from build123d import *

# Parameters (mm, degrees)
BOSS_EXTRU_1_DEPTH      = 20
ENL_V_MAT_EXTRU_1_DEPTH = 60.247890258
ESQUISSE5_W             = 53.8
ESQUISSE5_H             = 20
ESQUISSE5_R             = 3.2
ENL_V_MAT_EXTRU_2_DEPTH = 3
ESQUISSE6_W             = 53.8
ESQUISSE6_H             = 20
ESQUISSE6_R             = 6.75
ENL_V_MAT_EXTRU_3_DEPTH = 1.6
ESQUISSE7_W             = 53.8
ESQUISSE7_H             = 20
ENL_V_MAT_EXTRU_4_DEPTH = 3.2
CHANFREIN2_SIZE         = 3


with BuildPart() as part:
    # Esquisse1 → Boss.-Extru.1 (new body)
    with BuildSketch(Plane.XY):
        Polygon((0, 0), (40.1, 0), (40.1, 27.6), (46.95, 27.6), (46.95, 30.1), (40.1, 30.1), (40.1, 35.2), (36.7, 35.2), (36.7, 38.4), (16.402, 38.4), (16.402, 40), (12.852, 40), (12.852, 43), (6.452, 43), (6.452, 40), (2.902, 40), (2.902, 38.4), (0, 38.4), (0, 30.1), (-6.85, 30.1), (-6.85, 27.6), (0, 27.6), align=None)
    extrude(amount=BOSS_EXTRU_1_DEPTH)

    # Esquisse2 → Enlèv. mat.-Extru.1 (cut, through all)
    with BuildSketch(Plane(origin=(0, 30.1, 0), x_dir=(1, 0, 0), z_dir=(0, 1, 0))):
        with BuildLine():
            Line((-6.85, -3.75), (-6.85, -6.25))
            Line((-6.85, -6.25), (-6.186029115, -6.25))
            ThreePointArc((-6.186029115, -6.25), (-2.22, -5), (-6.186029115, -3.75))
            Line((-6.186029115, -3.75), (-6.85, -3.75))
        make_face()
        with BuildLine():
            Line((46.95, -6.25), (46.286029115, -6.25))
            ThreePointArc((46.286029115, -6.25), (42.32, -5), (46.286029115, -3.75))
            Line((46.286029115, -3.75), (46.95, -3.75))
            Line((46.95, -3.75), (46.95, -6.25))
        make_face()
        with BuildLine():
            Line((46.95, -16.25), (46.286029115, -16.25))
            ThreePointArc((46.286029115, -16.25), (42.32, -15), (46.286029115, -13.75))
            Line((46.286029115, -13.75), (46.95, -13.75))
            Line((46.95, -13.75), (46.95, -16.25))
        make_face()
        with BuildLine():
            Line((-6.85, -13.75), (-6.186029115, -13.75))
            ThreePointArc((-6.186029115, -13.75), (-2.22, -15), (-6.186029115, -16.25))
            Line((-6.186029115, -16.25), (-6.85, -16.25))
            Line((-6.85, -16.25), (-6.85, -13.75))
        make_face()
    extrude(amount=-ENL_V_MAT_EXTRU_1_DEPTH, mode=Mode.SUBTRACT)

    # Esquisse5 → Enlèv. mat.-Extru.2 (cut)
    with BuildSketch(Plane(origin=(0, 43, 0), x_dir=(1, 0, 0), z_dir=(0, 1, 0))):
        with Locations((20.05, -10)):
            Rectangle(ESQUISSE5_W, ESQUISSE5_H)
        with Locations(Location((9.652, -10, 0), (0, 0, 180))):
            Circle(ESQUISSE5_R, mode=Mode.SUBTRACT)
    extrude(amount=-ENL_V_MAT_EXTRU_2_DEPTH, mode=Mode.SUBTRACT)

    # Esquisse6 → Enlèv. mat.-Extru.3 (cut)
    with BuildSketch(Plane(origin=(0, 40, 0), x_dir=(1, 0, 0), z_dir=(0, 1, 0))):
        with Locations((20.05, -10)):
            Rectangle(ESQUISSE6_W, ESQUISSE6_H)
        with Locations(Location((9.652, -10, 0), (0, 0, 270))):
            Circle(ESQUISSE6_R, mode=Mode.SUBTRACT)
    extrude(amount=-ENL_V_MAT_EXTRU_3_DEPTH, mode=Mode.SUBTRACT)

    # Esquisse7 → Enlèv. mat.-Extru.4 (cut)
    with BuildSketch(Plane(origin=(0, 38.4, 0), x_dir=(1, 0, 0), z_dir=(0, 1, 0))):
        with Locations((20.05, -10)):
            Rectangle(ESQUISSE7_W, ESQUISSE7_H)
        with BuildLine():
            Line((13.446733192, -18.6), (36.7, -18.6))
            Line((36.7, -18.6), (36.7, -1.4))
            Line((36.7, -1.4), (13.446733192, -1.4))
            ThreePointArc((13.446733192, -1.4), (0.252, -10), (13.446733192, -18.6))
        make_face(mode=Mode.SUBTRACT)
    extrude(amount=-ENL_V_MAT_EXTRU_4_DEPTH, mode=Mode.SUBTRACT)

    # Chanfrein2
    chanfrein2_edges = [part.edges().sort_by_distance(p)[0] for p in [
        (36.7, 38.4, 10),
    ]]
    chamfer(chanfrein2_edges, length=CHANFREIN2_SIZE)


solid = part.part
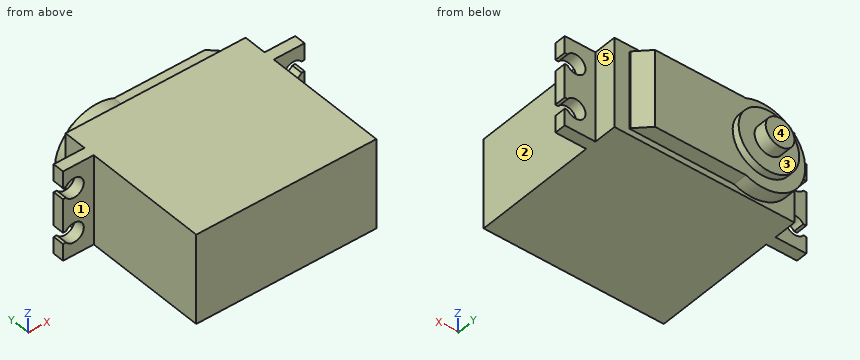
For this review, take the finished solid that the model builds, in its own axes (mm). Face numbers are marked on the shaded views. A direction names the side the tool comes from. Round coordinates to 2 decimals unless told otherwise and drop trailing zeros. Write each loop counter-clockwise with the first axis right and the second up, starting at its lowest first coordinate (ties: lowest second). Pieces come first, ordered by that corner, then holes. Notation, with made-up numbers: M 10.5,43.25 L 26.5,43.25 A20 cw 26.5,74.25 Z; hole C -31,9 d5. An arc over 180 degrees is marked long. Write item = value, one per line. Start each with the question number.
(1) We need section D-D (y = 7.5). Give the boundary of the cut face in (x, z).
(2) For line 1 along Z through (x, y) = (44.5, 29.35); line 2 along Z through (x, y) = (-4, 28); line 3 along X through (y, z) = (25, 18.75), list the stretches that pass through material, from the lowest coordinate up.
(3) We need section A-A (x = 44.5). Give the boundary of the cut face in (y, z).
(4) We need section B-B (z = 10). Give the boundary of the cut face in (x, y), then the cut area to 3 significant figures.
(5) We need section C-C (x = 23.5). Give the boundary of the cut face in (y, z), then the cut area to 3 significant figures.
(6) Clearance check with flat-ended pins moving along their axes: pin 1 Ø7 at (x, z) = (-4.4, 5) entering from +Y; pin 2 Ø1 at (x, y) = (26, 36.5) entering from +Z; pin 3 Ø1 at (x, z) = (18.5, 11.5) entering from +Y. State where each tip first meets the part, or that it passes through.
(7) For the marked faces 1, 2, 3, 4 and 5, list the 3-axis set-ups (+Z, -Z, +X, -X, +Y, -Y) from which the entire face can be reached by the end or side of a thin tool; tool diameter is ignored.
Results found:
q1.outline = M 0,0 L 40.1,0 L 40.1,20 L 0,20 Z
q2.line_1 = 0 to 2.82, 7.18 to 12.82, 17.18 to 20
q2.line_2 = 0 to 2.86, 7.14 to 12.86, 17.14 to 20
q2.line_3 = 0 to 40.1
q3.outline = M 27.6,0 L 30.1,0 L 30.1,2.82 L 27.6,2.82 Z; M 27.6,7.18 L 30.1,7.18 L 30.1,12.82 L 27.6,12.82 Z; M 27.6,17.18 L 30.1,17.18 L 30.1,20 L 27.6,20 Z
q4.outline = M -6.85,27.6 L 0,27.6 L 0,0 L 40.1,0 L 40.1,27.6 L 46.95,27.6 L 46.95,30.1 L 40.1,30.1 L 40.1,35.2 L 36.7,35.2 L 36.7,35.4 L 33.7,38.4 L 16.4,38.4 L 16.4,40 L 12.85,40 L 12.85,43 L 6.45,43 L 6.45,40 L 2.9,40 L 2.9,38.4 L 0.25,38.4 L 0.25,35.2 L 0,35.2 L 0,30.1 L -6.85,30.1 Z
q4.area = 1,600 mm²
q5.outline = M 0,0 L 35.2,0 L 35.2,1.4 L 38.4,1.4 L 38.4,18.6 L 35.2,18.6 L 35.2,20 L 0,20 Z
q5.area = 759 mm²
q6.pin_1 = 30.1
q6.pin_2 = 18.6
q6.pin_3 = 38.4
q7.face_1 = +Z, -Z, -X, -Y
q7.face_2 = +Z, -Z, +X, -Y
q7.face_3 = +Y
q7.face_4 = +Z, -Z, +X, -X, +Y
q7.face_5 = +Z, -Z, +X, +Y
